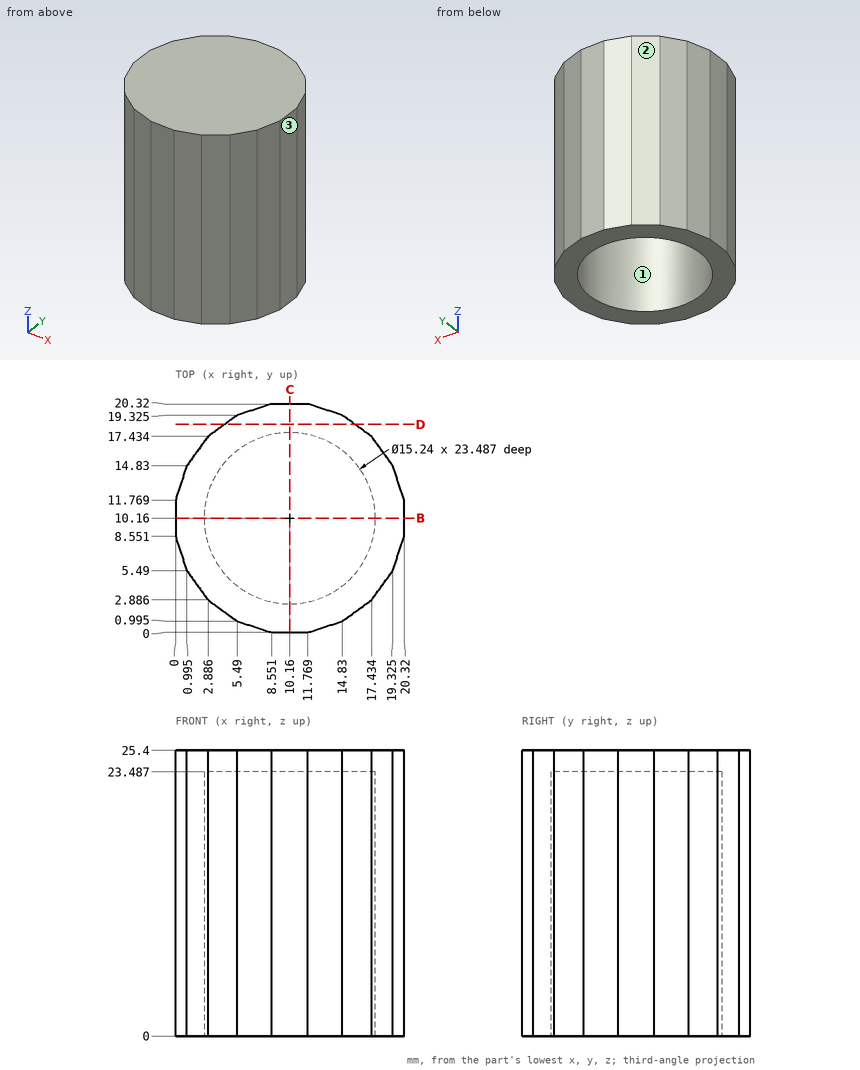
Job drawing, mm, ordinate dimensions from the low corner. One solid piece. Give positions to 0.01 mm unless a question says otherwise; leave off trailing zeros. Loops run counter-clockwise (first coordinate to the right, second up) from the corner with the lowest first, then second, coordinate; pieces in that order, holes last. Notation, with made-up numbers: (54.25, 58) -> (95.25, 58) arc R20 ccw to (95.25, 73) -> close; hole circle Ø5 at (-0.75, -36.5). An arc over 180 degrees is marked (long way). Use a Markdown table: item, result. Add a question column.
(1) Wall check: line 1 along Y through (x, z) = (10.16, 16.25); line 2 along X through (y, z) = (6, 14.75) (1 decimal); line 3 along X through (y, z) = (16.5, 22.5) (1 decimal). Give the ranges that are in metal, low to high.
(2) Slice it at D-D on y = 18.5. List the corners of the cut face in (x, z).
(3) Slice it at B-B on y = 10.16. List the corners of the cut face in (x, z).
(4) Drop flat-ended pins along their axis: pin 1 Ø10 at (x, z) = (17.5, 4.5) entering from +Y; pin 2 Ø8 at (y, z) = (4.5, 3) entering from -X; pin 3 Ø12 at (x, y) = (11, 10.5) entering from -Z. Give the stop position or say it passes through.
(5) Mould opens along X. For the marked faces 1, 2 and 3 say: +X half, -X half, draft (parallel to the pull), parting line (faces both ways), or undercut.
Filled sheet:
| question | item | result |
|---|---|---|
| 1 | line 1 | 0 to 2.54, 17.78 to 20.32 |
| 1 | line 2 | 0.8 to 3.8, 16.5 to 19.5 |
| 1 | line 3 | 2.2 to 5.9, 14.4 to 18.1 |
| 2 | outline | (4.35, 0) -> (15.97, 0) -> (15.97, 25.4) -> (4.35, 25.4) -> close |
| 3 | outline | (0, 0) -> (2.54, 0) -> (2.54, 23.49) -> (17.78, 23.49) -> (17.78, 0) -> (20.32, 0) -> (20.32, 25.4) -> (0, 25.4) -> close |
| 4 | pin 1 | y = 20.08 |
| 4 | pin 2 | x = 0.02 |
| 4 | pin 3 | z = 23.49 |
| 5 | face 1 | undercut |
| 5 | face 2 | -X half |
| 5 | face 3 | +X half |
